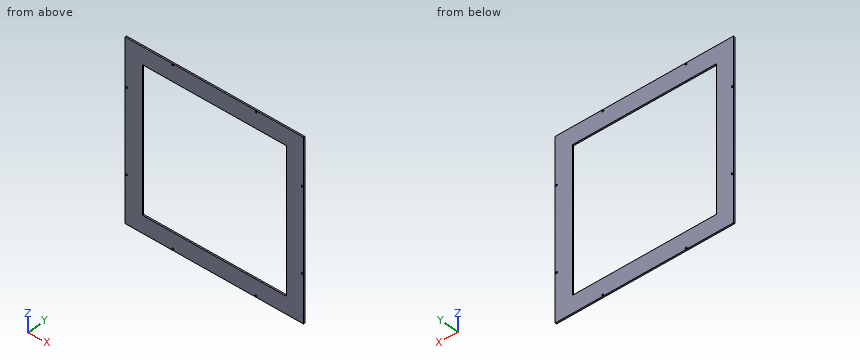
from build123d import *

# Parameters (mm, degrees)
SKETCH1_W           = 393.7
SKETCH1_H           = 393.7
BOSS_EXTRUDE1_DEPTH = 3.175
SKETCH2_W           = 317.5
SKETCH2_H           = 317.5
CUT_EXTRUDE1_DEPTH  = 279.40604452
SKETCH3_R           = 1.905
CUT_EXTRUDE3_DEPTH  = 279.40604452


with BuildPart() as part:
    # Sketch1 → Boss-Extrude1 (new body)
    with BuildSketch(Plane(origin=(0, 0, 0), x_dir=(1, 0, 0), z_dir=(0, 1, 0))):
        Rectangle(SKETCH1_W, SKETCH1_H)
    extrude(amount=BOSS_EXTRUDE1_DEPTH)

    # Sketch2 → Cut-Extrude1 (cut, through all)
    with BuildSketch(Plane(origin=(0, 3.175, 0), x_dir=(1, 0, 0), z_dir=(0, 1, 0))):
        Rectangle(SKETCH2_W, SKETCH2_H)
    extrude(amount=-CUT_EXTRUDE1_DEPTH, mode=Mode.SUBTRACT)

    # Sketch3 → Cut-Extrude3 (cut, through all)
    with BuildSketch(Plane(origin=(0, 3.175, 0), x_dir=(1, 0, 0), z_dir=(0, 1, 0))):
        with Locations(Location((-92.075, -193.675, 0), (0, 0, 270))):
            Circle(SKETCH3_R)
        with Locations(Location((92.075, -193.675, 0), (0, 0, 270))):
            Circle(SKETCH3_R)
        with Locations(Location((193.675, -92.075, 0), (0, 0, 270))):
            Circle(SKETCH3_R)
        with Locations(Location((193.675, 92.075, 0), (0, 0, 270))):
            Circle(SKETCH3_R)
        with Locations(Location((92.075, 193.675, 0), (0, 0, 270))):
            Circle(SKETCH3_R)
        with Locations(Location((-92.075, 193.675, 0), (0, 0, 270))):
            Circle(SKETCH3_R)
        with Locations(Location((-193.675, 92.075, 0), (0, 0, 270))):
            Circle(SKETCH3_R)
        with Locations(Location((-193.675, -92.075, 0), (0, 0, 270))):
            Circle(SKETCH3_R)
    extrude(amount=-CUT_EXTRUDE3_DEPTH, mode=Mode.SUBTRACT)


solid = part.part
The model under review builds one solid part; all positions refer to its coordinate system, in mm. Coordinates: 2 decimals unless noted, no trailing zeros. Loops run counter-clockwise (first coordinate to the right, second up) from the corner with the lowest first, then second, coordinate; pieces in that order, holes last. Notation, with made-up numbers: (64, 71) -> (88, 71) arc R27 cw to (88, 101) -> close; hole circle Ø2 at (69.25, -20.75). An arc over 180 degrees is marked (long way). Use a Markdown table: item, result. Add a question column.
1. Add section B-B on x = 20.5. Write out the cut boundary in (y, z) (3 decimals), plus the area to 3 significant figures.
2. To check wall thickness, follow line 1 (X direction, y = 2.25, z = -130). State the ranges of the line that lie inside material, in increasing order.
3. Add section C-C on y = 1.8. Give the number of separate pieces and of enclosed holes in the cut face, plus the area to 3 significant figures.
4. Add section A-A on z = -16.5. Write out the cut boundary in (x, y) (3 decimals), plus the area to 3 significant figures.
Returned:
| question | item | result |
|---|---|---|
| 1 | outline | (0, -196.85) -> (3.175, -196.85) -> (3.175, -158.75) -> (0, -158.75) -> close; (0, 158.75) -> (3.175, 158.75) -> (3.175, 196.85) -> (0, 196.85) -> close |
| 1 | area | 242 mm² |
| 2 | line 1 | x = -196.85 to -158.75, 158.75 to 196.85 |
| 3 | separate pieces | 1 |
| 3 | enclosed holes | 9 |
| 3 | area | 54,100 mm² |
| 4 | outline | (-196.85, 0) -> (-158.75, 0) -> (-158.75, 3.175) -> (-196.85, 3.175) -> close; (158.75, 0) -> (196.85, 0) -> (196.85, 3.175) -> (158.75, 3.175) -> close |
| 4 | area | 242 mm² |
